Here's the drawing with two shaded views (mm, measured from the low corner). I have some questions. A direction names the side the tool comes from. Round coordinates to 2 decimals unless told otherwise and drop trailing zeros. Order: outer loops, then holes, each group sorted by start corner. A loop starts at its lowest first (then second) coordinate and runs counter-clockwise, first axis right, second up.
Q1. For the marked faces 5 and 6, which set-ups out of +Z, -Z, +X, -X, +Y, -Y let a thin tool reach every point of the face, with its end or its side?
Q2. If we section it at C-C (z = 630): Please give me the cut outline in (x, y).
Q3. If I drill on line 1 (Y direction, x = 300, z = 56.5) (1 decimal); line 2 (Y direction, x = 344, z = 87) (1 decimal); line 3 (Z direction, x = 209, y = 106.5), over which ranges is the centre line in solid material (lowest first)?
Q4. We'd pull the mould along X, two halves only. Please class the marked faces 1, 2, 3 and 4: pulls with the +X half, pulls with the -X half, needs draft (parallel to the pull), parting line crosses it, or undercut.
Q5. If we section it at B-B (x = 300): Please give me the cut outline in (y, z) (1 decimal).
Q6. If we section it at D-D (x = 113.5): Please give me the cut outline in (y, z) (1 decimal), plus the area to 4 significant figures.
Q7. Will these pins go through, and if not, where does the flat tip stop? P1, Ø1, axis at x = 62, z = 558, coming from the -Y side; P2, Ø8, axis at x = 437.5, y = 207.5, coming from the -Z side; P3, Ø3, axis at x = 85, y = 811.5, coming from the +Z side.
Q8. If we section it at A-A (y = 250): Please give me the cut outline in (x, z), plus the area to 3 significant figures.
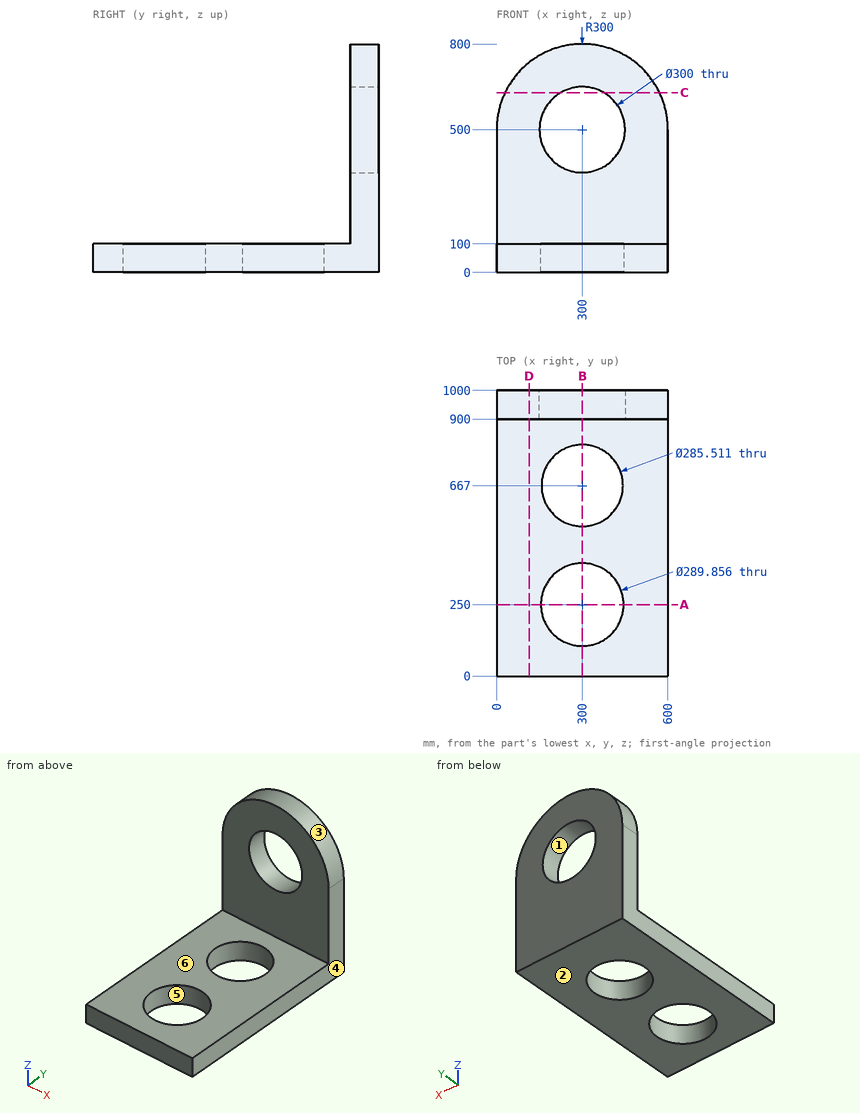
Solution:
1. face 5: +Z, -Z
1. face 6: +Z, +X, -X, -Y
2. outline: (29.63, 900) - (225.17, 900) - (225.17, 1000) - (29.63, 1000) - close; (374.83, 900) - (570.37, 900) - (570.37, 1000) - (374.83, 1000) - close
3. line 1: y = 0 to 105.1, 394.9 to 524.2, 809.8 to 1000
3. line 2: y = 0 to 111.9, 388.1 to 531.2, 802.8 to 1000
3. line 3: z = 0 to 100
4. face 1: undercut
4. face 2: needs draft
4. face 3: parting line crosses it
4. face 4: pulls with the +X half
5. outline: (0, 0) - (105.1, 0) - (105.1, 100) - (0, 100) - close; (394.9, 0) - (524.2, 0) - (524.2, 100) - (394.9, 100) - close; (809.8, 0) - (1000, 0) - (1000, 350) - (900, 350) - (900, 100) - (809.8, 100) - close; (900, 650) - (1000, 650) - (1000, 800) - (900, 800) - close
6. outline: (0, 0) - (1000, 0) - (1000, 735) - (900, 735) - (900, 100) - (0, 100) - close
6. area: 163,500 mm2
7. P1: stops at y = 900
7. P2: stops at z = 0
7. P3: stops at z = 100
8. outline: (0, 0) - (155.07, 0) - (155.07, 100) - (0, 100) - close; (444.93, 0) - (600, 0) - (600, 100) - (444.93, 100) - close
8. area: 31,000 mm2
